Part model, mm, in its own coordinate system. Face numbers are marked on the shaded views. A direction names the side the tool comes from. Coordinates: 2 decimals unless noted, no trailing zeros. Order: outer loops, then holes, each group sorted by start corner. A loop starts at its lowest first (then second) coordinate and runs counter-clockwise, first axis right, second up.
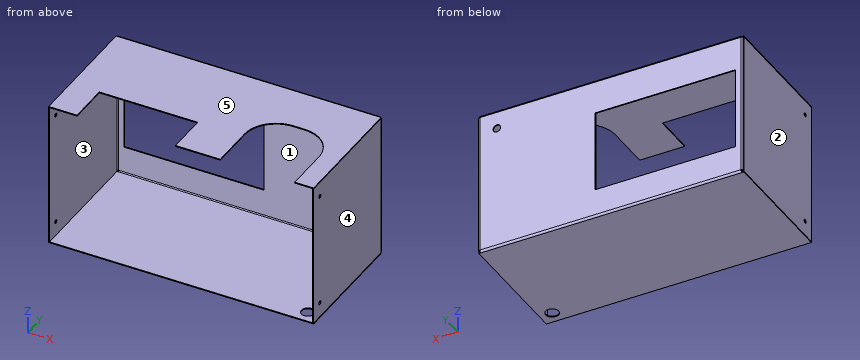
from build123d import *

# Parameters (mm, degrees)
BASE_FLANGE2_DEPTH       = 210
SKETCH8_R                = 6
SKETCH8_W                = 222
SKETCH8_H                = 130
CUT_EXTRUDE1_DEPTH       = 10
SKETCH14_W               = 156
SKETCH14_H               = 65
SKETCH14_W_2             = 118
SKETCH14_H_2             = 121
CUT_EXTRUDE2_DEPTH       = 10
EDGE_FLANGE1_START       = -115
EDGE_FLANGE1_DEPTH       = 230
EDGE_FLANGE1_2_DEPTH     = 3
EDGE_FLANGE1_START_2     = 112
EDGE_FLANGE1_3_DEPTH     = 3
EDGE_FLANGE1_START_3     = -112
EDGE_FLANGE1_4_DEPTH     = 224
CLOSED_START             = -129.163047535
CLOSED_CORNER1_OUTLINE_W = 1.5
CLOSED_CORNER1_OUTLINE_H = 1.4
CLOSED_CORNER1_DEPTH     = 197
SKETCH35_R               = 10.25
CUT_EXTRUDE4_DEPTH       = 210
FILLET1_R                = 50
SKETCH37_R               = 3
CUT_EXTRUDE5_DEPTH       = 580


# Read off the part's stored shape, not the designer's step: Edge-Flange1, Closed Corner1
# Sheet-metal steps are written as plain solids
with BuildPart() as part:
    # Sketch5 → Base-Flange2 (new, symmetric)
    with BuildSketch(Plane(origin=(0, 0, 0), x_dir=(0, 0, -1), z_dir=(1, 0, 0))):
        with BuildLine():
            Line((-115, -129.163047535), (-115, 67.836952465))
            ThreePointArc((-115, 67.836952465), (-114.121320344, 69.958272808), (-112, 70.836952465))
            Line((-112, 70.836952465), (112, 70.836952465))
            ThreePointArc((112, 70.836952465), (114.121320344, 69.958272808), (115, 67.836952465))
            Line((115, 67.836952465), (115, -129.163047535))
            Line((115, -129.163047535), (113.5, -129.163047535))
            Line((113.5, -129.163047535), (113.5, 67.836952465))
            ThreePointArc((113.5, 67.836952465), (113.060660172, 68.897612636), (112, 69.336952465))
            Line((112, 69.336952465), (-112, 69.336952465))
            ThreePointArc((-112, 69.336952465), (-113.060660172, 68.897612636), (-113.5, 67.836952465))
            Line((-113.5, 67.836952465), (-113.5, -129.163047535))
            Line((-113.5, -129.163047535), (-115, -129.163047535))
        make_face()
    extrude(amount=BASE_FLANGE2_DEPTH, both=True)

    # Sketch8 → Cut-Extrude1 (cut)
    with BuildSketch(Plane(origin=(0, 70.836952465, 0), x_dir=(1, 0, 0), z_dir=(0, 1, 0))):
        with Locations(Location((180, -85, 0), (0, 0, 270))):
            Circle(SKETCH8_R)
        with Locations((-87, 5)):
            Rectangle(SKETCH8_W, SKETCH8_H)
    extrude(amount=-CUT_EXTRUDE1_DEPTH, mode=Mode.SUBTRACT)

    # Sketch14 → Cut-Extrude2 (cut)
    with BuildSketch(Plane.XY.offset(115)):
        with Locations((-87, -96.663047535)):
            Rectangle(SKETCH14_W, SKETCH14_H)
        with Locations((121, -68.663047535)):
            Rectangle(SKETCH14_W_2, SKETCH14_H_2)
    extrude(amount=-CUT_EXTRUDE2_DEPTH, mode=Mode.SUBTRACT)

    # Edge-Flange1 outline → Edge-Flange1 (cut)
    with BuildSketch(Plane.XY.offset(EDGE_FLANGE1_START)):
        with BuildLine():
            Line((210, 67.836952465), (210, 70.836952465))
            Line((210, 70.836952465), (207, 70.836952465))
            ThreePointArc((207, 70.836952465), (209.121320344, 69.958272808), (210, 67.836952465))
        make_face()
        with BuildLine():
            Line((207, 67.836952465), (208.5, 67.836952465))
            ThreePointArc((208.5, 67.836952465), (208.060660172, 68.897612636), (207, 69.336952465))
            Line((207, 69.336952465), (207, 67.836952465))
        make_face()
        with BuildLine():
            Line((-207, 67.836952465), (-207, 69.336952465))
            ThreePointArc((-207, 69.336952465), (-208.060660172, 68.897612636), (-208.5, 67.836952465))
            Line((-208.5, 67.836952465), (-207, 67.836952465))
        make_face()
        with BuildLine():
            Line((-207, 70.836952465), (-210, 70.836952465))
            Line((-210, 70.836952465), (-210, 67.836952465))
            ThreePointArc((-210, 67.836952465), (-209.121320344, 69.958272808), (-207, 70.836952465))
        make_face()
    extrude(amount=EDGE_FLANGE1_DEPTH, mode=Mode.SUBTRACT)

    # Edge-Flange1 2 outline → Edge-Flange1 2 (cut)
    with BuildSketch(Plane.XY.offset(EDGE_FLANGE1_START)):
        with BuildLine():
            Line((208.5, 67.836952465), (210, 67.836952465))
            ThreePointArc((210, 67.836952465), (209.121320344, 69.958272808), (207, 70.836952465))
            Line((207, 70.836952465), (207, 69.336952465))
            ThreePointArc((207, 69.336952465), (208.060660172, 68.897612636), (208.5, 67.836952465))
        make_face()
        with BuildLine():
            ThreePointArc((-207, 70.836952465), (-209.121320344, 69.958272808), (-210, 67.836952465))
            Line((-210, 67.836952465), (-208.5, 67.836952465))
            ThreePointArc((-208.5, 67.836952465), (-208.060660172, 68.897612636), (-207, 69.336952465))
            Line((-207, 69.336952465), (-207, 70.836952465))
        make_face()
    extrude(amount=EDGE_FLANGE1_2_DEPTH, mode=Mode.SUBTRACT)

    # Edge-Flange1 3 outline → Edge-Flange1 3 (cut)
    with BuildSketch(Plane.XY.offset(EDGE_FLANGE1_START_2)):
        with BuildLine():
            Line((208.5, 67.836952465), (210, 67.836952465))
            ThreePointArc((210, 67.836952465), (209.121320344, 69.958272808), (207, 70.836952465))
            Line((207, 70.836952465), (207, 69.336952465))
            ThreePointArc((207, 69.336952465), (208.060660172, 68.897612636), (208.5, 67.836952465))
        make_face()
        with BuildLine():
            ThreePointArc((-207, 70.836952465), (-209.121320344, 69.958272808), (-210, 67.836952465))
            Line((-210, 67.836952465), (-208.5, 67.836952465))
            ThreePointArc((-208.5, 67.836952465), (-208.060660172, 68.897612636), (-207, 69.336952465))
            Line((-207, 69.336952465), (-207, 70.836952465))
        make_face()
    extrude(amount=EDGE_FLANGE1_3_DEPTH, mode=Mode.SUBTRACT)

    # Edge-Flange1 4 outline → Edge-Flange1 4 (add)
    with BuildSketch(Plane.XY.offset(EDGE_FLANGE1_START_3)):
        with BuildLine():
            Line((210, -129.163047535), (210, 67.836952465))
            ThreePointArc((210, 67.836952465), (209.897777479, 68.6134096), (209.598076211, 69.336952465))
            Line((209.598076211, 69.336952465), (207, 69.336952465))
            ThreePointArc((207, 69.336952465), (208.060660172, 68.897612636), (208.5, 67.836952465))
            Line((208.5, 67.836952465), (208.5, -129.163047535))
            Line((208.5, -129.163047535), (210, -129.163047535))
        make_face()
        with BuildLine():
            ThreePointArc((-208.5, 67.836952465), (-208.060660172, 68.897612636), (-207, 69.336952465))
            Line((-207, 69.336952465), (-209.598076211, 69.336952465))
            ThreePointArc((-209.598076211, 69.336952465), (-209.897777479, 68.6134096), (-210, 67.836952465))
            Line((-210, 67.836952465), (-210, -129.163047535))
            Line((-210, -129.163047535), (-208.5, -129.163047535))
            Line((-208.5, -129.163047535), (-208.5, 67.836952465))
        make_face()
    extrude(amount=EDGE_FLANGE1_4_DEPTH)

    # Closed Corner1 outline → Closed Corner1 (add)
    with BuildSketch(Plane(origin=(0, 0, 0), x_dir=(1, 0, 0), z_dir=(0, 1, 0)).offset(CLOSED_START)):
        with Locations((-209.25, -112.7)):
            Rectangle(CLOSED_CORNER1_OUTLINE_W, CLOSED_CORNER1_OUTLINE_H)
        with Locations((-209.25, 112.7)):
            Rectangle(CLOSED_CORNER1_OUTLINE_W, CLOSED_CORNER1_OUTLINE_H)
        with Locations((209.25, -112.7)):
            Rectangle(CLOSED_CORNER1_OUTLINE_W, CLOSED_CORNER1_OUTLINE_H)
        with Locations((209.25, 112.7)):
            Rectangle(CLOSED_CORNER1_OUTLINE_W, CLOSED_CORNER1_OUTLINE_H)
    extrude(amount=CLOSED_CORNER1_DEPTH)

    # Sketch35 → Cut-Extrude4 (cut)
    with BuildSketch(Plane(origin=(95, 0, -115), x_dir=(1, 0, 0), z_dir=(0, 0, 1))):
        with Locations(Location((95, -109.163047535, 0), (0, 0, 270))):
            Circle(SKETCH35_R)
    extrude(amount=CUT_EXTRUDE4_DEPTH, mode=Mode.SUBTRACT)

    # Fillet1
    fillet1_edges = [part.edges().sort_by_distance(p)[0] for p in [
        (180, -8.163047535, 114.25),
        (62, -8.163047535, 114.25),
    ]]
    fillet(fillet1_edges, radius=FILLET1_R)

    # Sketch37 → Cut-Extrude5 (cut)
    with BuildSketch(Plane(origin=(210, 0, 0), x_dir=(0, 0, -1), z_dir=(1, 0, 0))):
        with Locations(Location((-90, -111.163047535, 0), (0, 0, 90))):
            Circle(SKETCH37_R)
        with Locations(Location((90, -111.163047535, 0), (0, 0, 270))):
            Circle(SKETCH37_R)
    extrude(amount=-CUT_EXTRUDE5_DEPTH, mode=Mode.SUBTRACT)


solid = part.part
Q1. Wall check: line 1 along X through (y, z) = (40, -6); line 2 along Z through (x, y) = (-23, 4.5); line 3 along Y through (x, z) = (-209.6, -90). Give the ranges that are in metal, low to high.
Results list:
line 1: x = -210 to -208.5, 208.5 to 210
line 2: z = -115 to -113.5, 113.5 to 115
line 3: y = -129.16 to -114.16, -108.16 to 69.33
Q2. Pin check, flat tips, straight feed: pin 1 Ø0.8 at (x, z) = (-208.5, -114.5) entering from +Y; pin 2 Ø12 at (x, z) = (49, -68) entering from -Y; pin 3 Ø1.2 at (y, z) = (70, -9) entering from -X. Stop position of each tip, or through.
Results list:
pin 1: stops at y = 67.84
pin 2: stops at y = 69.34
pin 3: stops at x = -209.56
Q3. Which spindle directions (+Z, -Z, +X, -X, +Y, -Y) get a long thin tool onto all of the face, cutting with end or side? Do the marked faces 1 and 2. Say none if no direction does.
Results list:
face 1: -Y
face 2: +Z, -Z, -X, +Y, -Y
Q4. Mould opens along X. For the marked faces 3, 4 and 5 say: pulls with the +X half, pulls with the -X half, needs draft (parallel to the pull), parting line crosses it, or undercut.
Results list:
face 3: undercut
face 4: pulls with the +X half
face 5: needs draft
Q5. Cut at D-D on y = -74. Write the cut outline in (x, z), and give its area (3 significant figures).
Results list:
outline: (-210, -115) - (210, -115) - (210, -113.5) - (-210, -113.5) - close; (-210, -113.4) - (-208.5, -113.4) - (-208.5, 113.4) - (-210, 113.4) - close; (-210, 113.5) - (-165, 113.5) - (-165, 115) - (-210, 115) - close; (-9, 113.5) - (62, 113.5) - (62, 115) - (-9, 115) - close; (180, 113.5) - (210, 113.5) - (210, 115) - (180, 115) - close; (208.5, -113.4) - (210, -113.4) - (210, 113.4) - (208.5, 113.4) - close
area: 1,530 mm2
Q6. Cut at C-C on x = -113. Write the cut outline in (y, z).
Results list:
outline: (-129.16, -115) - (67.84, -115) arc R3 ccw to (70.84, -112) - (70.84, -70) - (69.34, -70) - (69.34, -112) arc R1.5 cw to (67.84, -113.5) - (-129.16, -113.5) - close; (-64.16, 113.5) - (67.84, 113.5) arc R1.5 cw to (69.34, 112) - (69.34, 60) - (70.84, 60) - (70.84, 112) arc R3 ccw to (67.84, 115) - (-64.16, 115) - close
Q7. Cut at B-B on z = -12. Write the cut outline in (x, y), and give its area (3 significant figures).
Results list:
outline: (-210, -129.16) - (-208.5, -129.16) - (-208.5, 67.84) arc R1.5 cw to (-207, 69.34) - (-198, 69.34) - (-198, 70.84) - (-207, 70.84) arc R3 ccw to (-210, 67.84) - close; (24, 69.34) - (207, 69.34) arc R1.5 cw to (208.5, 67.84) - (208.5, -129.16) - (210, -129.16) - (210, 67.84) arc R3 ccw to (207, 70.84) - (24, 70.84) - close
area: 890 mm2
Q8. Cut at A-A on y = 18. Write the cut outline in (x, z).
Results list:
outline: (-210, -115) - (210, -115) - (210, -113.5) - (-210, -113.5) - close; (-210, -113.4) - (-208.5, -113.4) - (-208.5, 113.4) - (-210, 113.4) - close; (-210, 113.5) - (210, 113.5) - (210, 115) - (-210, 115) - close; (208.5, -113.4) - (210, -113.4) - (210, 113.4) - (208.5, 113.4) - close
